from build123d import *

# Parameters (mm, degrees)
SKETCH_1_W           = 95
SKETCH_1_H           = 62
EXTRUDE_1_DEPTH      = 2
EXTRUDE_2_DEPTH      = 15
EXTRUDE_2_DEPTH_BACK = 77
SKETCH_2_R           = 16
FILLET_1_R           = 5
CUT_EXTRUDE_START    = -3
SKETCH_3_R           = 13
CUT_EXTRUDE_3_DEPTH  = 106.341404828
SKETCH_5_R           = 6
CUT_EXTRUDE_4_DEPTH  = 106.805765438


with BuildPart() as part:
    # 草图1 → 凸台-拉伸1 (new body)
    with BuildSketch(Plane.XY):
        Rectangle(SKETCH_1_W, SKETCH_1_H)
        with BuildLine():
            Line((-39.5, 26.65), (-35.5, 26.65))
            ThreePointArc((-35.5, 26.65), (-31.35, 22.5), (-35.5, 18.35))
            Line((-35.5, 18.35), (-39.5, 18.35))
            ThreePointArc((-39.5, 18.35), (-43.65, 22.5), (-39.5, 26.65))
        make_face(mode=Mode.SUBTRACT)
        with BuildLine():
            Line((39.5, 26.65), (35.5, 26.65))
            ThreePointArc((35.5, 26.65), (31.35, 22.5), (35.5, 18.35))
            Line((35.5, 18.35), (39.5, 18.35))
            ThreePointArc((39.5, 18.35), (43.65, 22.5), (39.5, 26.65))
        make_face(mode=Mode.SUBTRACT)
        with BuildLine():
            Line((-39.5, -26.65), (-35.5, -26.65))
            ThreePointArc((-35.5, -26.65), (-31.35, -22.5), (-35.5, -18.35))
            Line((-35.5, -18.35), (-39.5, -18.35))
            ThreePointArc((-39.5, -18.35), (-43.65, -22.5), (-39.5, -26.65))
        make_face(mode=Mode.SUBTRACT)
        with BuildLine():
            Line((39.5, -26.65), (35.5, -26.65))
            ThreePointArc((35.5, -26.65), (31.35, -22.5), (35.5, -18.35))
            Line((35.5, -18.35), (39.5, -18.35))
            ThreePointArc((39.5, -18.35), (43.65, -22.5), (39.5, -26.65))
        make_face(mode=Mode.SUBTRACT)
    extrude(amount=EXTRUDE_1_DEPTH)

    # 草图2 → 凸台-拉伸2 (add, two sides: drawn at the far end of the back side and taken through both)
    with BuildSketch(Plane(origin=(0, 31, 0), x_dir=(1, 0, 0), z_dir=(0, 1, 0)).offset(-EXTRUDE_2_DEPTH_BACK)):
        with Locations(Location((0, 15.9, 0), (0, 0, 180))):
            Circle(SKETCH_2_R)
    extrude(amount=EXTRUDE_2_DEPTH + EXTRUDE_2_DEPTH_BACK)

    # 圆角1
    fillet_1_edges = [part.edges().sort_by_distance(p)[0] for p in [
        (-47.5, 31, 1),
        (47.5, 31, 1),
        (47.5, -31, 1),
        (-47.5, -31, 1),
    ]]
    fillet(fillet_1_edges, radius=FILLET_1_R)

    # 草图3 → 切除-拉伸3 (cut, through all)
    with BuildSketch(Plane(origin=(0, 46, 0), x_dir=(1, 0, 0), z_dir=(0, 1, 0)).offset(CUT_EXTRUDE_START)):
        with Locations(Location((0, 15.9, 0), (0, 0, 180))):
            Circle(SKETCH_3_R)
    extrude(amount=-CUT_EXTRUDE_3_DEPTH, mode=Mode.SUBTRACT)

    # 草图5 → 切除-拉伸4 (cut, through all)
    with BuildSketch(Plane(origin=(0, 43, 0), x_dir=(-1, 0, 0), z_dir=(0, -1, 0))):
        with Locations(Location((0, 15.9, 0), (0, 0, 180))):
            Circle(SKETCH_5_R)
    extrude(amount=-CUT_EXTRUDE_4_DEPTH, mode=Mode.SUBTRACT)


solid = part.part
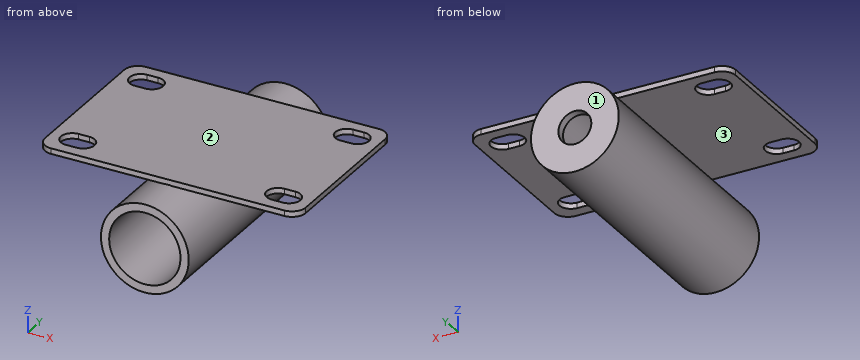
Geometry check sheet. Reference: the model listing, model coordinates, mm. Face numbers are marked on the shaded views. Round coordinates to 2 decimals unless told otherwise and drop trailing zeros. Order: outer loops, then holes, each group sorted by start corner. A loop starts at its lowest first (then second) coordinate and runs counter-clockwise, first axis right, second up. Notation, with made-up numbers: (-24, 60) -> (11, 60) arc R19 cw to (11, 93) -> close; hole circle Ø8 at (2.25, 16.25). An arc over 180 degrees is marked (long way). Use one line per item in the form item = value.
1. Mould release check, pull along Z, two halves, no side actions. Record for the marked faces 1, 2 and 3: pulls with the +Z half, pulls with the -Z half, needs draft (parallel to the pull), parting line crosses it, or undercut.
Working result:
face_1 = needs draft
face_2 = pulls with the +Z half
face_3 = undercut
2. Scan lines: line 1 along Z through (x, y) = (0, 44); line 2 along Z through (x, y) = (0, -4); line 3 along Z through (x, y) = (8.5, -19). Record each from-to range of solid material in increasing order. Write a range as from..to.
Working result:
line_1 = -31.9..-21.9, -9.9..0.1
line_2 = -31.9..-28.9, -2.9..2
line_3 = -29.46..-25.74, -6.06..-2.34, 0..2
3. Cross-section at D-D, the plane x = 0. Enter the section's corners in (y, z).
Working result:
outline = (-46, -31.9) -> (46, -31.9) -> (46, -21.9) -> (43, -21.9) -> (43, -28.9) -> (-46, -28.9) -> close; (-46, -2.9) -> (43, -2.9) -> (43, -9.9) -> (46, -9.9) -> (46, 0.1) -> (31, 0.1) -> (31, 2) -> (-31, 2) -> (-31, 0.1) -> (-46, 0.1) -> close
4. Cross-section at B-B, the plane z = -15.9. Enter the section's corners in (x, y).
Working result:
outline = (-16, -46) -> (-13, -46) -> (-13, 43) -> (-6, 43) -> (-6, 46) -> (-16, 46) -> close; (6, 43) -> (13, 43) -> (13, -46) -> (16, -46) -> (16, 46) -> (6, 46) -> close
5. Cross-section at C-C, the plane y = -3. Enter the section's corners in (x, z), plus the area to 3 significant figures.
Working result:
outline = (-47.5, 0) -> (-1.79, 0) arc R16 ccw (long way) to (1.79, 0) -> (47.5, 0) -> (47.5, 2) -> (-47.5, 2) -> close; hole circle Ø26 at (0, -15.9)
area = 463 mm^2
6. Go/stop test with flat-tipped pins: pin 1 (1 mm diameter, centred on x = -37.5, z = 1.5, fed in from +Y); pin 2 (0.6 mm diameter, centred on x = -37, z = 1.5, fed in from -Y); pin 3 (8 mm diameter, centred on x = 1.5, z = -18, fed in from -Y); pin 4 (12 mm diameter, centred on x = -22.5, z = -11, fed in from -Y). Record where each tip stops, or that it passes through.
Working result:
pin_1 = 31
pin_2 = -31
pin_3 = 43
pin_4 = through
7. Cross-section at A-A, the plane y = 22.5. Enter the section's corners in (x, z).
Working result:
outline = (-47.5, 0) -> (-43.65, 0) -> (-43.65, 2) -> (-47.5, 2) -> close; (-31.35, 0) -> (-1.79, 0) arc R16 ccw (long way) to (1.79, 0) -> (31.35, 0) -> (31.35, 2) -> (-31.35, 2) -> close; (43.65, 0) -> (47.5, 0) -> (47.5, 2) -> (43.65, 2) -> close; hole circle Ø26 at (0, -15.9)
